Here's how the part is built. I have some questions about the finished solid (model axes, mm). A direction names the side the tool comes from. Round coordinates to 2 decimals unless told otherwise and drop trailing zeros. Loops run counter-clockwise (first coordinate to the right, second up) from the corner with the lowest first, then second, coordinate; pieces in that order, holes last. Notation, with made-up numbers: M -37,10.5 L -17,10.5 A22 cw -17,46.5 Z; hole C 69,72.25 d5. An arc over 180 degrees is marked long. Answer as a JSON object with one key per item and string values.
Autodesk Inventor part; units mm, degrees
ref_plane "YZ Plane" through (0, 0, 0) normal (1, 0, 0) x (0, 1, 0)
ref_plane "XZ Plane" through (0, 0, 0) normal (0, 1, 0) x (-1, 0, 0)
ref_plane "XY Plane" through (0, 0, 0) normal (0, 0, 1) x (1, 0, 0)
sketch "スケッチ1" plane through (0, 0, 0) normal (0, 0, 1) x (1, 0, 0)
  line L0 (18, -18) -> (-18, -18)
  line L1 (-18, -18) -> (-18, 18)
  line L2 (-18, 18) -> (18, 18)
  line L3 (18, 18) -> (18, -18)
  line L4 (18, -18) -> (-18, 18) construction
  line L5 (-18, -18) -> (18, 18) construction
  point P0 (0, 0)
  point P1 (0, 0)
  dimension "d34" = 36
  dimension "d35" = 36
extrude "押し出し1" add sketch "スケッチ1" along normal blind 4
sketch "スケッチ3" plane through (0, 0, 4) normal (0, 0, 1) x (1, 0, 0)
  line L0 (-9, -5.5) -> (9, -5.5)
  line L1 (9, -5.5) -> (9, 5.5)
  line L2 (9, 5.5) -> (-9, 5.5)
  line L3 (-9, 5.5) -> (-9, -5.5)
  line L4 (-9, -5.5) -> (9, 5.5) construction
  line L5 (9, -5.5) -> (-9, 5.5) construction
  point P0 (0, 0)
  dimension "d18" = 18
  dimension "d19" = 11
hole "穴2" at (-9, 5.5, 4) at (-9, -5.5, 4) at (9, -5.5, 4) at (9, 5.5, 4) direction (0, 0, -1) diameter 3.3 end through all
sketch "スケッチ4" plane through (0, 0, 4) normal (0, 0, 1) x (1, 0, 0)
  circle A0 centre (0, 0) radius 8.5
  dimension "d27" = 17
extrude "押し出し2" cut sketch "スケッチ4" against normal through all
sketch "スケッチ5" plane through (0, 0, 4) normal (0, 0, 1) x (1, 0, 0)
  circle A0 centre (0, 0) radius 15
  point P0 (0, 15)
  point P1 (-15, 0)
  point P2 (0, -15)
  point P3 (15, 0)
  dimension "d36" = 30
  dimension "d39" = 360
hole "穴3" at (15, 0, 4) at (-15, 0, 4) at (0, 15, 4) direction (0, 0, -1) diameter 3.2 end through all
sketch "スケッチ6" plane through (0, 0, 4) normal (0, 0, 1) x (1, 0, 0)
  circle A0 centre (0, 0) radius 16
  point P0 (-11.3137, 11.3137)
  point P1 (-11.3137, -11.3137)
  point P2 (11.3137, -11.3137)
  point P3 (11.3137, 11.3137)
  dimension "d48" = 32
  dimension "d51" = 360
hole "穴4" at (-11.3137, 11.3137, 4) at (-11.3137, -11.3137, 4) at (11.3137, -11.3137, 4) at (11.3137, 11.3137, 4) direction (0, 0, -1) diameter 4.3 end through all counterbore diameter 7.6 counterbore depth 10
sketch "スケッチ9" plane through (0, 0, 4) normal (0, 0, 1) x (1, 0, 0)
  line L0 (-11, -7.5) -> (11, -7.5)
  line L1 (11, -7.5) -> (11, 7.5)
  line L2 (11, 7.5) -> (-11, 7.5)
  line L3 (-11, 7.5) -> (-11, -7.5)
  line L4 (-11, -7.5) -> (11, 7.5) construction
  line L5 (11, -7.5) -> (-11, 7.5) construction
  line L6 (-18, 18) -> (-18, -18)
  line L7 (-18, -7.5) -> (18, -7.5)
  line L8 (18, -7.5) -> (18, -18)
  line L9 (18, -18) -> (-18, -18)
  line L10 (-18, -18) -> (-18, -7.5)
  line L11 (18, -18) -> (18, 18)
  point P0 (0, 0)
  point P1 (18, -11.3137)
  point P2 (18, 11.3137)
  point P3 (-18, -11.3137)
  dimension "d71" = 22
  dimension "d72" = 15
extrude "押し出し5" cut sketch "スケッチ9" against normal through all contours L0 L7 L8 L9 L6
fillet "フィレット2" radius 2 4 edges at (4, -7.5, 2) (-4, -7.5, 2) (-18, -7.5, 2) (18, -7.5, 2)
sketch "スケッチ11" plane through (0, 0, 0) normal (0, 0, -1) x (-1, 0, 0)
  point P0 (0, 0)
fillet "フィレット4" radius 6.6865 2 edges at (-18, 18, 2) (18, 18, 2)
properties part number "unit-base5" material "ABS プラスチック"
Item 1: If we mould it in two halves opening along X, with no side actions, what happens to faces 3 (the face through (12, -7.5, 2)), 4 (the face through (12.769, 7.803, 1.972)), 5 (the face through (-18, 3, 2))? For each: pulls with the +X half, pulls with the -X half, needs draft (parallel to the pull), parting line crosses it, or undercut.
Resolved:
{"face 3": "needs draft", "face 4": "undercut", "face 5": "pulls with the -X half"}
Item 2: I want a section at D-D, the plane y = 5.5. Please give me the cut outline in (x, z).
Resolved:
{"outline": "M -18,0 L -10.65,0 L -10.65,4 L -18,4 Z; M -7.35,0 L -6.48,0 L -6.48,4 L -7.35,4 Z; M 6.48,0 L 7.35,0 L 7.35,4 L 6.48,4 Z; M 10.65,0 L 18,0 L 18,4 L 10.65,4 Z"}
Item 3: I'm going to push flat-ended pins straight in: pin 1 Ø2.5 at (x, y) = (-15, 0) entering from +Z; pin 2 Ø1 at (y, z) = (14.5, 0.5) entering from -X. Where does each tip first touch, or does it pass through?
Resolved:
{"pin 1": "through", "pin 2": "x = -17.44"}
Item 4: I want a section at C-C, the plane x = 14.5. Please give me the cut outline in (y, z), then the cut area to 3 significant figures.
Resolved:
{"outline": "M -7.5,0 L -1.52,0 L -1.52,4 L -7.5,4 Z; M 1.52,0 L 9.24,0 L 9.24,4 L 1.52,4 Z; M 13.38,0 L 17.19,0 L 17.19,4 L 13.38,4 Z", "area": "70.0 mm²"}
Item 5: I want a section at B-B, the plane y = -3. Please give me the cut outline in (x, z), then the cut area to 3 significant figures.
Resolved:
{"outline": "M -18,0 L -7.95,0 L -7.95,4 L -18,4 Z; M 7.95,0 L 18,0 L 18,4 L 7.95,4 Z", "area": "80.4 mm²"}
Item 6: On a 3-axis mill with a long thin cutter (end or side, diameter ignored), from which of +Z, -Z, +X, -X, +Y, -Y can I reach the whole of each face in a straight line? I mean faces 1 (the face through (-13, -7.5, 2)), 2 (the face through (7.184, -6.45, 2.028)). Say none if no direction works.
Resolved:
{"face 1": "+Z, -Z, +X, -X, -Y", "face 2": "+Z, -Z"}
Item 7: Please list where these lines run through material, in increasing order: probe 1 along X at (y, z) = (0, 2.6); probe 2 along Y at (x, z) = (-14, 0.25); probe 3 along Y at (x, z) = (0, 1.55). Write a range as from..to.
Resolved:
{"probe 1": "-18..-16.6, -13.4..-8.5, 8.5..13.4, 16.6..18", "probe 2": "-7.5..-1.25, 1.25..8.63, 14..17.44", "probe 3": "8.5..13.4, 16.6..18"}
Item 8: I want a section at A-A, the plane x = 9.5. Please give me the cut outline in (y, z), then the cut area to 3 significant figures.
Resolved:
{"outline": "M -7.5,0 L -7.07,0 L -7.07,4 L -7.5,4 Z; M -3.93,0 L 3.93,0 L 3.93,4 L -3.93,4 Z; M 7.07,0 L 7.97,0 L 7.97,4 L 7.07,4 Z; M 14.65,0 L 18,0 L 18,4 L 14.65,4 Z", "area": "50.1 mm²"}
